from build123d import *

# Parameters (mm, degrees)
SKETCH2_R          = 4
SKETCH2_R_2        = 3
BASE_FLANGE1_DEPTH = 3.175
FILLET1_R          = 2


# Sheet-metal steps are written as plain solids
with BuildPart() as part:
    # Sketch2 → Base-Flange1 (new body)
    with BuildSketch(Plane.XZ.offset(-47.844717124)):
        Polygon((208.087093798, -67.18067292), (208.087093798, -37.24408426), (193.087093798, -37.24408426), (193.087093798, -52.18067292), (137.087093798, -52.18067292), (137.087093798, -67.18067292), align=None)
        with Locations(Location((147.087093798, -59.257788189, 0), (0, 0, 270))):
            Circle(SKETCH2_R, mode=Mode.SUBTRACT)
        with Locations(Location((200.587093798, -43.757788189, 0), (0, 0, 270))):
            Circle(SKETCH2_R_2, mode=Mode.SUBTRACT)
    extrude(amount=BASE_FLANGE1_DEPTH)

    # Fillet1
    fillet1_edges = [part.edges().sort_by_distance(p)[0] for p in [
        (193.087093798, 46.257217124, -37.24408426),
        (208.087093798, 46.257217124, -37.24408426),
        (208.087093798, 46.257217124, -67.18067292),
        (137.087093798, 46.257217124, -67.18067292),
        (137.087093798, 46.257217124, -52.18067292),
    ]]
    fillet(fillet1_edges, radius=FILLET1_R)


solid = part.part
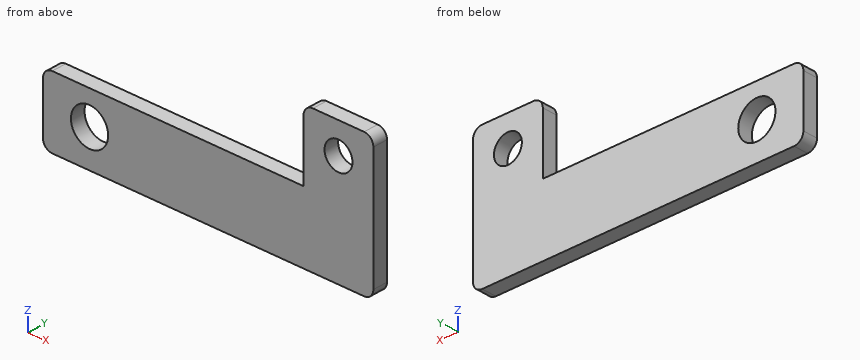
Can you work these out from the model? Positions are in its coordinate system, mm. Coordinates: 2 decimals unless noted, no trailing zeros. Order: outer loops, then holes, each group sorted by start corner. A loop starts at its lowest first (then second) coordinate and runs counter-clockwise, first axis right, second up. Notation, with made-up numbers: (-20, -36.5) -> (1, -36.5) arc R18 cw to (1, -32.5) -> close; hole circle Ø9 at (-4, 86.25). An arc over 180 degrees is marked (long way). Use one line per item in the form item = value.
Q1. Imagine slicing it at D-D, the plane x = 176. List the corners of the cut face in (y, z) for me, then the cut area to 3 significant figures.
From the geometry:
outline = (44.67, -67.18) -> (47.84, -67.18) -> (47.84, -52.18) -> (44.67, -52.18) -> close
area = 47.6 mm²
Q2. Will these pins go through, and if not, where does the flat tip stop? P1, Ø1, axis at y = 45.5, z = -49, coming from the -X side; P2, Ø5, axis at x = 200.59, z = -43.76, coming from the -Y side.
From the geometry:
P1 = 193.09
P2 = through
Q3. I need wall thicknesses on L1, parallel to Z at x = 177.5, y = 45.65; L2, parallel to X at y = 47.5, z = -42.5; L3, parallel to X at y = 47.6, z = -54. Which ranges of each line are inside material? Lowest first, please.
From the geometry:
L1 = -67.18 to -52.18
L2 = 193.09 to 197.86, 203.31 to 208.09
L3 = 137.1 to 208.09
Q4. Imagine slicing it at B-B, the plane y = 45.45. List the corners of the cut face in (x, z) for me, then the cut area to 3 significant figures.
From the geometry:
outline = (137.09, -65.18) arc R2 ccw to (139.09, -67.18) -> (206.09, -67.18) arc R2 ccw to (208.09, -65.18) -> (208.09, -39.24) arc R2 ccw to (206.09, -37.24) -> (195.09, -37.24) arc R2 ccw to (193.09, -39.24) -> (193.09, -52.18) -> (139.09, -52.18) arc R2 ccw to (137.09, -54.18) -> close; hole circle Ø8 at (147.09, -59.26); hole circle Ø6 at (200.59, -43.76)
area = 1,210 mm²
Q5. Imagine slicing it at C-C, the plane z = -42.75. List the corners of the cut face in (x, y) for me, then the cut area to 3 significant figures.
From the geometry:
outline = (193.09, 44.67) -> (197.76, 44.67) -> (197.76, 47.84) -> (193.09, 47.84) -> close; (203.41, 44.67) -> (208.09, 44.67) -> (208.09, 47.84) -> (203.41, 47.84) -> close
area = 29.7 mm²
Q6. Imagine slicing it at A-A, the plane z = -59.25. List the corners of the cut face in (x, y) for me.
From the geometry:
outline = (137.09, 44.67) -> (143.09, 44.67) -> (143.09, 47.84) -> (137.09, 47.84) -> close; (151.09, 44.67) -> (208.09, 44.67) -> (208.09, 47.84) -> (151.09, 47.84) -> close
